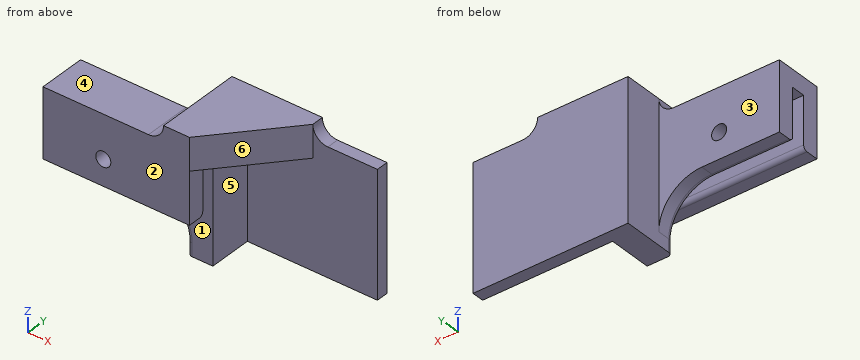
```python
from build123d import *

# Parameters (mm, degrees)
SKETCH_1_W          = 34
SKETCH_1_H          = 16
EXTRUDE_1_DEPTH     = 11
SKETCH_2_W          = 34
SKETCH_2_H          = 3.2
CUT_EXTRUDE_1_DEPTH = 12
HOLE_WIZARD_1_D     = 3.5
SKETCH_6_W          = 6
SKETCH_6_H          = 3.9
EXTRUDE_2_DEPTH     = 13
FILLET_1_R          = 10
SKETCH_7_W          = 6
SKETCH_7_H          = 29
EXTRUDE_3_DEPTH     = 9
SKETCH_8_W          = 29
SKETCH_8_H          = 2.8
EXTRUDE_4_DEPTH     = 30
EXTRUDE_6_DEPTH     = 3.5
FILLET_2_R          = 1
FILLET_3_R          = 3.5
FILLET_4_R          = 3.5
EXTRUDE_7_DEPTH     = 4
SKETCH_12_W         = 0.2
SKETCH_12_H         = 10.1
CUT_EXTRUDE_2_DEPTH = 25


# Some blends are built 0.0001 mm under size
with BuildPart() as part:
    # 草图1 → 凸台-拉伸1 (new body)
    with BuildSketch(Plane(origin=(0, 0, 0), x_dir=(1, 0, 0), z_dir=(0, 1, 0))):
        with Locations((17, -8)):
            Rectangle(SKETCH_1_W, SKETCH_1_H)
    extrude(amount=EXTRUDE_1_DEPTH)

    # 草图2 → 切除-拉伸1 (cut)
    with BuildSketch(Plane(origin=(0, 0, 0), x_dir=(-1, 0, 0), z_dir=(0, 0, -1))):
        with Locations((-17, 5.5)):
            Rectangle(SKETCH_2_W, SKETCH_2_H)
    extrude(amount=-CUT_EXTRUDE_1_DEPTH, mode=Mode.SUBTRACT)

    # 孔1 (through all)
    with Locations(Plane(origin=(0, 11, 0), x_dir=(1, 0, 0), z_dir=(0, 1, 0))):
        with Locations((14, -6)):
            Hole(HOLE_WIZARD_1_D / 2)

    # 草图6 → 凸台-拉伸2 (add)
    with BuildSketch(Plane(origin=(0, 0, 0), x_dir=(-1, 0, 0), z_dir=(0, 0, -1))):
        with Locations((-31, 9.05)):
            Rectangle(SKETCH_6_W, SKETCH_6_H)
    extrude(amount=EXTRUDE_2_DEPTH)

    # 圆角1
    fillet_1_edges = [part.edges().sort_by_distance(p)[0] for p in [
        (28, 9.05, 0),
    ]]
    fillet(fillet_1_edges, radius=FILLET_1_R)

    # 草图7 → 凸台-拉伸3 (add)
    with BuildSketch(Plane(origin=(0, 11, 0), x_dir=(1, 0, 0), z_dir=(0, 1, 0))):
        with Locations((31, -1.5)):
            Rectangle(SKETCH_7_W, SKETCH_7_H)
    extrude(amount=EXTRUDE_3_DEPTH)

    # 草图8 → 凸台-拉伸4 (add)
    with BuildSketch(Plane(origin=(34, 0, 0), x_dir=(0, 0, -1), z_dir=(1, 0, 0))):
        with Locations((-1.5, 18.6)):
            Rectangle(SKETCH_8_W, SKETCH_8_H)
    extrude(amount=EXTRUDE_4_DEPTH)

    # 草图10 → 凸台-拉伸6 (add)
    with BuildSketch(Plane.XY.offset(16)):
        Polygon((28, 0), (34, 0), (34, 17.2), (49, 17.2), (49, 20), (28, 20), (28, 11), align=None)
        Polygon((34, 17.2), (34, 0), (49, 17.2), align=None)
    extrude(amount=EXTRUDE_6_DEPTH)

    # 圆角2
    fillet_2_edges = [part.edges().sort_by_distance(p)[0] for p in [
        (9, 7.1, 0),
        (17, 3.9, 0),
        (28, 7.1, -11.5),
        (25.071067812, 7.1, -2.928932188),
    ]]
    fillet(fillet_2_edges, radius=FILLET_2_R)

    # 圆角3
    fillet_3_edges = [part.edges().sort_by_distance(p)[0] for p in [
        (28, 5.5, 16),
    ]]
    fillet(fillet_3_edges, radius=FILLET_3_R - 0.0001)  # a hair under: the kernel refuses the full size

    # 圆角4
    # the kernel refuses this fillet: 3.5 mm, written as the material it adds along each edge
    with BuildSketch(Plane(origin=(49, 17.2, 16), x_dir=(0, 0, 1), z_dir=(0, 1, 0))) as fillet_4_piece_1:
        with BuildLine():
            CenterArc((FILLET_4_R, FILLET_4_R), FILLET_4_R, 180, 90)
            Line((0, FILLET_4_R), (0, 0))
            Line((0, 0), (FILLET_4_R, 0))
        make_face()
    extrude(amount=2.8)

    # 草图11 → 凸台-拉伸7 (add)
    with BuildSketch(Plane(origin=(0, 0, 16), x_dir=(-1, 0, 0), z_dir=(0, 0, -1))):
        Polygon((-49, 17.2), (-34, 17.2), (-34, 0), align=None)
    extrude(amount=EXTRUDE_7_DEPTH)

    # 草图12 → 切除-拉伸2 (cut)
    with BuildSketch(Plane(origin=(0, 0, -13), x_dir=(-1, 0, 0), z_dir=(0, 0, -1))):
        with Locations((-33.9, 12.15)):
            Rectangle(SKETCH_12_W, SKETCH_12_H)
    extrude(amount=-CUT_EXTRUDE_2_DEPTH, mode=Mode.SUBTRACT)


solid = part.part
```
Work out the finished part from the listing and answer in its coordinate system (mm). Face numbers are marked on the shaded views. A direction names the side the tool comes from. Round coordinates to 2 decimals unless told otherwise and drop trailing zeros. Write each loop counter-clockwise with the first axis right and the second up, starting at its lowest first coordinate (ties: lowest second). Pieces come first, ordered by that corner, then holes.
1) Flat-ended cylindrical pins translate along their axes: P1, Ø2, axis at y = 13, z = 13, coming from the +X side; P2, Ø12, axis at x = 7, z = -3, coming from the +Y side; P3, Ø1, axis at x = 7.5, y = 4.5, coming from the -Z side; P4, Ø10, axis at y = 2, z = -9, coming from the -X side. Find the tip coordinate at first contact, or state that the pin passes through.
2) A cutting plane is placed at C-C on z = 2.5. Determine the outline of the cut face in (x, y).
3) A cutting plane is placed at A-A on z = 6. Determine the outline of the cut face in (x, y).
4) A cutting plane is placed at B-B on x = 14. Determine the outline of the cut face in (y, z).
5) Which of the six approach directions +Z, -Z, +X, -X, +Y, -Y give full straight-line access (tool end or side, diameter ignored) to the marked faces 1, 2 and 3?
6) Determine the mould class of the marked faces 4, 5 and 6 for opening direction Y: pulls with the +Y half, pulls with the -Y half, needs draft (parallel to the pull), parting line crosses it, or undercut.
7) Consider probe 1 along Z at (x, y) = (14, 2.2); probe 2 along X at (y, z) = (1.85, 6); probe 3 along X at (y, z) = (9.05, 6). Determine where each line is inside the solid, lowest interval first.
Entries:
1. P1: stops at x = 46.21
1. P2: stops at y = 11
1. P3: stops at z = 12
1. P4: passes through
2. outline: (0, 0) - (34, 0) - (34, 3.9) - (0, 3.9) - close; (0, 7.1) - (33.8, 7.1) - (33.8, 17.2) - (64, 17.2) - (64, 20) - (28, 20) - (28, 11) - (0, 11) - close
3. outline: (0, 0) - (12.25, 0) - (12.25, 3.9) - (0, 3.9) - close; (0, 7.1) - (12.25, 7.1) - (12.25, 11) - (0, 11) - close; (15.75, 0) - (34, 0) - (34, 3.9) - (15.75, 3.9) - close; (15.75, 7.1) - (33.8, 7.1) - (33.8, 17.2) - (64, 17.2) - (64, 20) - (28, 20) - (28, 11) - (15.75, 11) - close
4. outline: (0, 0) - (2.9, 0) arc R1 ccw to (3.9, 1) - (3.9, 4.25) - (0, 4.25) - close; (0, 7.75) - (3.9, 7.75) - (3.9, 12) - (7.1, 12) - (7.1, 7.75) - (11, 7.75) - (11, 16) - (0, 16) - close; (7.1, 1) arc R1 ccw to (8.1, 0) - (11, 0) - (11, 4.25) - (7.1, 4.25) - close
5. face 1: -Z, +X, -X
5. face 2: +Z, -Z, +X, -X, -Y
5. face 3: +Z, -Z, -X, +Y
6. face 4: needs draft
6. face 5: undercut
6. face 6: pulls with the -Y half
7. probe 1: z = 0 to 4.25, 7.75 to 16
7. probe 2: x = 0 to 12.25, 15.75 to 34
7. probe 3: x = 0 to 12.25, 15.75 to 33.8
